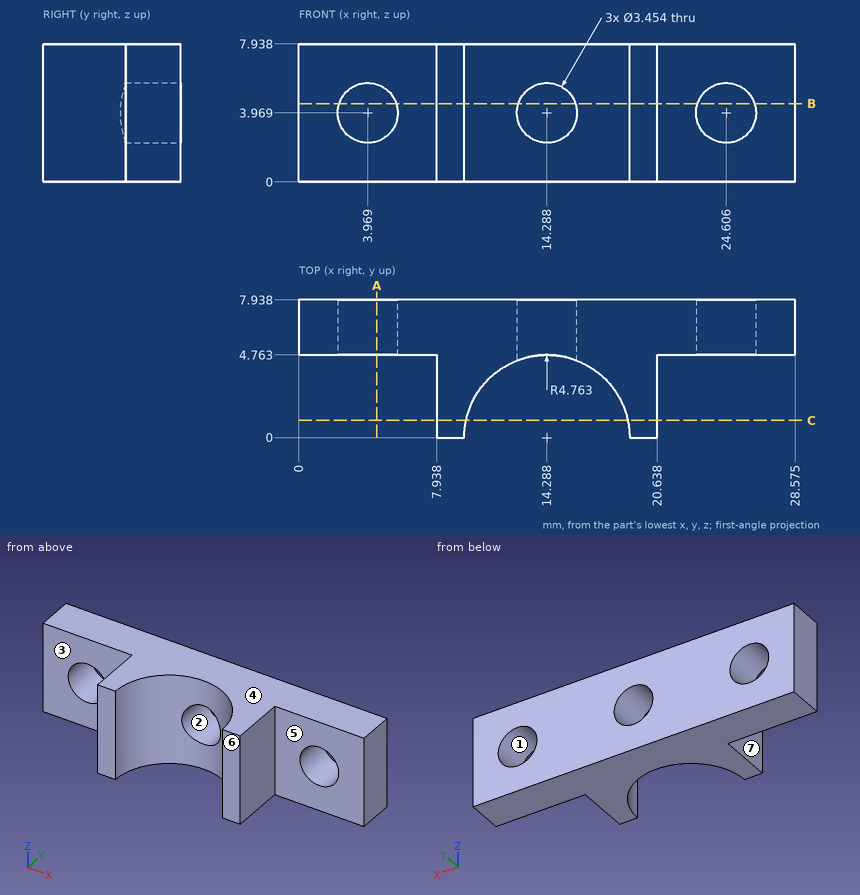
Print and shaded views of the part. All mm, measured from the part's lowest x, y and z. A direction names the side the tool comes from. Coordinates: 2 decimals unless noted, no trailing zeros. Loops run counter-clockwise (first coordinate to the right, second up) from the corner with the lowest first, then second, coordinate; pieces in that order, holes last. Notation, with made-up numbers: (18, -11) -> (35, -11) arc R37 cw to (35, 26) -> close; hole circle Ø7 at (5, -37.75). An arc over 180 degrees is marked (long way). Use one line per item in the form item = value. Start each with the question number.
(1) Cut at A-A on x = 4.5. Give the cut face in (y, z) (1 decimal).
(2) Cut at B-B on z = 4.5. Give the number of separate pieces and of enclosed holes in the cut face.
(3) Probe probe 1 along X at (y, z) = (5.25, 3) (1 decimal); probe 2 along X at (y, z) = (6.75, 4.75) (1 decimal); probe 3 along Y at (x, z) = (22, 3.25). List the from-to ranges inside material, lowest first. Write a range as from..to.
(4) Flat gauge pins, fed straight in: pin 1 (3 mm diameter, centred on x = 14.29, z = 3.97, fed in from -Y); pin 2 (4.5 mm diameter, centred on x = 24.61, z = 3.97, fed in from -Y); pin 3 (1.4 mm diameter, centred on y = 2, z = 2, fed in from -X); pin 4 (4 mm diameter, centred on y = 1.5, z = 3, fed in from +X). Where does each tip first touch, or does it go through?
(5) Pull direction Z, two halves, no side cores. Call the marked faces 1, 2, 3 and 4: pulls with the +Z half, pulls with the -Z half, needs draft (parallel to the pull), parting line crosses it, or undercut.
(6) Tool access for the marked faces 5, 6 and 7: list every direction of +Z, -Z, +X, -X, +Y, -Y with a clear straight run to the whole face (end or side of a thin tool).
(7) Cut at C-C on y = 1. Give the cut face in (x, z).
Values:
q1.outline = (4.8, 0) -> (7.9, 0) -> (7.9, 2.3) -> (4.8, 2.3) -> close; (4.8, 5.6) -> (7.9, 5.6) -> (7.9, 7.9) -> (4.8, 7.9) -> close
q2.separate_pieces = 4
q2.enclosed_holes = 0
q3.probe_1 = 0..2.5, 5.4..12.9, 15.7..23.2, 26..28.6
q3.probe_2 = 0..2.4, 5.5..12.7, 15.8..23.1, 26.1..28.6
q3.probe_3 = 4.76..7.94
q4.pin_1 = through
q4.pin_2 = 4.76
q4.pin_3 = 7.94
q4.pin_4 = 20.64
q5.face_1 = undercut
q5.face_2 = undercut
q5.face_3 = needs draft
q5.face_4 = pulls with the +Z half
q6.face_5 = +Z, -Z, +X, -Y
q6.face_6 = +Z, -Z, +X, -X, -Y
q6.face_7 = +Z, -Z, -X, -Y
q7.outline = (7.94, 0) -> (9.63, 0) -> (9.63, 7.94) -> (7.94, 7.94) -> close; (18.94, 0) -> (20.64, 0) -> (20.64, 7.94) -> (18.94, 7.94) -> close
